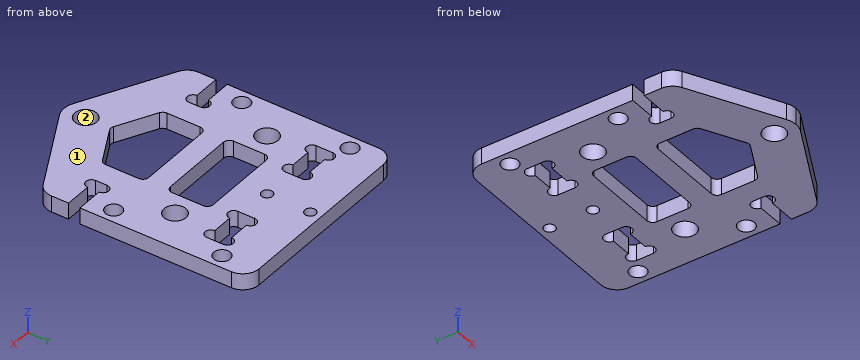
from build123d import *

# Parameters (mm, degrees)
SKETCH_1_W          = 38.4
SKETCH_1_H          = 47.5
SKETCH_1_R          = 2.025
EXTRUDE_1_DEPTH     = 3
SKETCH_2_R          = 1.025
CUT_EXTRUDE_1_DEPTH = 43
SKETCH_3_W          = 7.1
SKETCH_3_H          = 2.1
CUT_EXTRUDE_2_DEPTH = 3
CUT_EXTRUDE_3_DEPTH = 3
SKETCH_5_R          = 1.525
CUT_EXTRUDE_4_DEPTH = 3
SKETCH_6_W          = 8.1
SKETCH_6_H          = 3.1
CUT_EXTRUDE_5_DEPTH = 3
SKETCH_7_R          = 1.05
CUT_EXTRUDE_6_DEPTH = 3
CUT_EXTRUDE_7_DEPTH = 3
FILLET_1_R          = 3
SKETCH_9_W          = 16
SKETCH_9_H          = 7.89799579
CUT_EXTRUDE_8_DEPTH = 3
FILLET_2_R          = 1.1


with BuildPart() as part:
    # 草图1 → 凸台-拉伸1 (new body)
    with BuildSketch(Plane.XY):
        with Locations((0, 7.25)):
            Rectangle(SKETCH_1_W, SKETCH_1_H)
        with Locations((-12, 12.5)):
            Circle(SKETCH_1_R, mode=Mode.SUBTRACT)
        with Locations((12, 12.5)):
            Circle(SKETCH_1_R, mode=Mode.SUBTRACT)
        with Locations((0, -12.5)):
            Circle(SKETCH_1_R, mode=Mode.SUBTRACT)
    extrude(amount=EXTRUDE_1_DEPTH)

    # 草图2 → 切除-拉伸1 (cut)
    with BuildSketch(Plane(origin=(0, 0, 0), x_dir=(-1, 0, 0), z_dir=(0, 0, -1))):
        with Locations((0, 29)):
            Circle(SKETCH_2_R)
        with Locations((0, 21)):
            Circle(SKETCH_2_R)
    extrude(amount=-CUT_EXTRUDE_1_DEPTH, mode=Mode.SUBTRACT)

    # 草图3 → 切除-拉伸2 (cut)
    with BuildSketch(Plane.XY.offset(3)):
        with Locations((15.7, -1)):
            Rectangle(SKETCH_3_W, SKETCH_3_H)
        with Locations((-15.7, -1)):
            Rectangle(SKETCH_3_W, SKETCH_3_H)
    extrude(amount=-CUT_EXTRUDE_2_DEPTH, mode=Mode.SUBTRACT)

    # 草图4 → 切除-拉伸3 (cut)
    with BuildSketch(Plane.XY.offset(3)):
        with BuildLine():
            ThreePointArc((-12.15, -2.05), (-12.45753788, -1.30753788), (-13.2, -1))
            ThreePointArc((-13.2, -1), (-13.94246212, -1.30753788), (-14.25, -2.05))
            Line((-14.25, -2.05), (-12.15, -2.05))
        make_face()
        with BuildLine():
            ThreePointArc((-14.25, -2.05), (-13.2, -3.1), (-12.15, -2.05))
            Line((-12.15, -2.05), (-14.25, -2.05))
        make_face()
        with BuildLine():
            Line((-14.25, 0.05), (-12.15, 0.05))
            ThreePointArc((-12.15, 0.05), (-13.2, 1.1), (-14.25, 0.05))
        make_face()
        with BuildLine():
            ThreePointArc((-13.2, -1), (-12.45753788, -0.69246212), (-12.15, 0.05))
            Line((-12.15, 0.05), (-14.25, 0.05))
            ThreePointArc((-14.25, 0.05), (-13.94246212, -0.69246212), (-13.2, -1))
        make_face()
        with BuildLine():
            ThreePointArc((14.25, -2.05), (13.94246212, -1.30753788), (13.2, -1))
            ThreePointArc((13.2, -1), (12.45753788, -1.30753788), (12.15, -2.05))
            Line((12.15, -2.05), (14.25, -2.05))
        make_face()
        with BuildLine():
            ThreePointArc((12.15, -2.05), (13.2, -3.1), (14.25, -2.05))
            Line((14.25, -2.05), (12.15, -2.05))
        make_face()
        with BuildLine():
            Line((12.15, 0.05), (14.25, 0.05))
            ThreePointArc((14.25, 0.05), (13.2, 1.1), (12.15, 0.05))
        make_face()
        with BuildLine():
            ThreePointArc((13.2, -1), (13.94246212, -0.69246212), (14.25, 0.05))
            Line((14.25, 0.05), (12.15, 0.05))
            ThreePointArc((12.15, 0.05), (12.45753788, -0.69246212), (13.2, -1))
        make_face()
    extrude(amount=-CUT_EXTRUDE_3_DEPTH, mode=Mode.SUBTRACT)

    # 草图5 → 切除-拉伸4 (cut)
    with BuildSketch(Plane(origin=(0, 0, 0), x_dir=(-1, 0, 0), z_dir=(0, 0, -1))):
        with Locations((16.7, 4.5)):
            Circle(SKETCH_5_R)
        with Locations((16.7, 24.5)):
            Circle(SKETCH_5_R)
        with Locations((-16.7, 24.5)):
            Circle(SKETCH_5_R)
        with Locations((-16.7, 4.5)):
            Circle(SKETCH_5_R)
    extrude(amount=-CUT_EXTRUDE_4_DEPTH, mode=Mode.SUBTRACT)

    # 草图6 → 切除-拉伸5 (cut)
    with BuildSketch(Plane.XY.offset(3)):
        with Locations((-10.2, 21.5)):
            Rectangle(SKETCH_6_W, SKETCH_6_H)
    cut_extrude_5 = extrude(amount=-CUT_EXTRUDE_5_DEPTH, mode=Mode.SUBTRACT)

    # 草图7 → 切除-拉伸6 (cut)
    with BuildSketch(Plane.XY.offset(3)):
        with Locations((-13.2, 19.95)):
            Circle(SKETCH_7_R)
        with Locations((-13.2, 23.05)):
            Circle(SKETCH_7_R)
        with Locations((-7.2, 23.05)):
            Circle(SKETCH_7_R)
        with Locations((-7.2, 19.95)):
            Circle(SKETCH_7_R)
    cut_extrude_6 = extrude(amount=-CUT_EXTRUDE_6_DEPTH, mode=Mode.SUBTRACT)

    # 镜向1: 切除-拉伸5, 切除-拉伸6 across plane
    add(cut_extrude_5.mirror(Plane(origin=(0, 0, 0), x_dir=(0, 0, 1), z_dir=(1, 0, 0))), mode=Mode.SUBTRACT)
    add(cut_extrude_6.mirror(Plane(origin=(0, 0, 0), x_dir=(0, 0, 1), z_dir=(1, 0, 0))), mode=Mode.SUBTRACT)

    # 草图8 → 切除-拉伸7 (cut)
    with BuildSketch(Plane.XY.offset(3)):
        with BuildLine():
            Line((-19.2, -16.5), (0, -16.5))
            ThreePointArc((0, -16.5), (-0.947626647, -16.38612966), (-1.84130001, -16.051001869))
            Line((-1.84130001, -16.051001869), (-19.2, -7.05))
            Line((-19.2, -7.05), (-19.2, -16.5))
        make_face()
        with BuildLine():
            Line((19.2, -7.05), (1.84130001, -16.051001869))
            ThreePointArc((1.84130001, -16.051001869), (0.947626647, -16.38612966), (0, -16.5))
            Line((0, -16.5), (19.2, -16.5))
            Line((19.2, -16.5), (19.2, -7.05))
        make_face()
    extrude(amount=-CUT_EXTRUDE_7_DEPTH, mode=Mode.SUBTRACT)

    # 圆角1
    fillet_1_edges = [part.edges().sort_by_distance(p)[0] for p in [
        (-19.2, -7.05, 1.5),
        (19.2, -7.05, 1.5),
        (-19.2, 31, 1.5),
        (19.2, 31, 1.5),
    ]]
    fillet(fillet_1_edges, radius=FILLET_1_R)

    # 草图9 → 切除-拉伸8 (cut)
    with BuildSketch(Plane(origin=(0, 0, 0), x_dir=(-1, 0, 0), z_dir=(0, 0, -1))):
        Polygon((8, 4.05200421), (-8, 4.05200421), (-8, -3.845991579), (0, -7.99422935), (8, -3.845991579), align=None)
        with Locations((0, 12.001002105)):
            Rectangle(SKETCH_9_W, SKETCH_9_H)
    extrude(amount=-CUT_EXTRUDE_8_DEPTH, mode=Mode.SUBTRACT)

    # 圆角2
    fillet_2_edges = [part.edges().sort_by_distance(p)[0] for p in [
        (8, -3.845991579, 1.5),
        (0, -7.99422935, 1.5),
        (-8, -3.845991579, 1.5),
        (-8, 4.05200421, 1.5),
        (8, 4.05200421, 1.5),
        (-8, 8.05200421, 1.5),
        (-8, 15.95, 1.5),
        (8, 15.95, 1.5),
        (8, 8.05200421, 1.5),
    ]]
    fillet(fillet_2_edges, radius=FILLET_2_R)


solid = part.part
Geometry: final body of the model. Coordinates: model frame, mm. Face numbers are marked on the shaded views. Round coordinates to 2 decimals unless told otherwise and drop trailing zeros. Order: outer loops, then holes, each group sorted by start corner. A loop starts at its lowest first (then second) coordinate and runs counter-clockwise, first axis right, second up. Notation, with made-up numbers: (89, 50) -> (120, 50) arc R17 cw to (120, 65) -> close; hole circle Ø2 at (4, -4.75). An arc over 180 degrees is marked (long way). Put each result on its own line as item: value. Start each with the question number.
Q1. Pull-direction query (Y, two-part tool) for the marked faces 1 and 2; classes: +Y half, -Y half, draft (parallel to the pull), parting line (faces both ways), or undercut.
Q2. Section A-A on x = -13.5. Return the cut outline in (y, z).
Q3. Section C-C on z = 1.9. Give the number of separate pieces and of enclosed holes in the cut face, and give its area (3 significant figures).
Q4. First-contact query: pin 1 (4.5 mm diameter, centred on x = 0, y = -12.5, fed in from +Z); pin 2 (1.5 mm diameter, centred on x = -4, z = 0.5, fed in from -Y). Flat tips, straight axial feed; report the tip coordinate or a pass-through.
Q5. Line query: probe 1 along Y at (x, z) = (0, 2.4) (3 decimals); probe 2 along Y at (x, z) = (16.7, 1.75) (3 decimals); probe 3 along Y at (x, z) = (-12, 0.8) (3 decimals). Output: solid intervals per line, ascending.
Q6. Section D-D on x = -9. Return the cut outline in (y, z), and give its area (3 significant figures).
Q7. Section B-B on x = 3. Return the cut outline in (y, z).
Ans:
1. face 1: draft
1. face 2: undercut
2. outline: (-10.01, 0) -> (-3.06, 0) -> (-3.06, 3) -> (-10.01, 3) -> close; (1.06, 0) -> (11.14, 0) -> (11.14, 3) -> (1.06, 3) -> close; (13.86, 0) -> (18.94, 0) -> (18.94, 3) -> (13.86, 3) -> close; (24.06, 0) -> (31, 0) -> (31, 3) -> (24.06, 3) -> close
3. separate pieces: 1
3. enclosed holes: 13
3. area: 1,190 mm2
4. pin 1: stops at z = 3
4. pin 2: stops at y = -15.32
5. probe 1: y = -16.5 to -14.525, -10.475 to -7.855, 4.052 to 8.052, 15.95 to 19.975, 22.025 to 27.975, 30.025 to 31
5. probe 2: y = -8.346 to -2.05, 0.05 to 2.975, 6.025 to 22.975, 26.025 to 30.958
5. probe 3: y = -10.783 to 10.475, 14.525 to 19.95, 23.05 to 31
6. outline: (-12.34, 0) -> (19.95, 0) -> (19.95, 3) -> (-12.34, 3) -> close; (23.05, 0) -> (31, 0) -> (31, 3) -> (23.05, 3) -> close
6. area: 121 mm2
7. outline: (-15.45, 0) -> (-6.44, 0) -> (-6.44, 3) -> (-15.45, 3) -> close; (4.05, 0) -> (8.05, 0) -> (8.05, 3) -> (4.05, 3) -> close; (15.95, 0) -> (31, 0) -> (31, 3) -> (15.95, 3) -> close
